```python
from build123d import *

# Parameters (mm, degrees)
SM_BASE_FLANGE_3_DEPTH = 50
SKETCH_14_R            = 6
SKETCH_14_R_2          = 1.5
CUT_EXTRUDE_1_DEPTH    = 69.26602376
SKETCH_15_R            = 2
CUT_EXTRUDE_2_DEPTH    = 94.257707456
FILLET_1_R             = 5


# Sheet-metal steps are written as plain solids
with BuildPart() as part:
    # 草图1 → 基体-法兰3 (new body)
    with BuildSketch(Plane(origin=(0, 0, 0), x_dir=(1, 0, 0), z_dir=(0, 1, 0))):
        with BuildLine():
            Line((-35.5, 34), (-35.5, 6))
            ThreePointArc((-35.5, 6), (-33.742640687, 1.757359313), (-29.5, 0))
            Line((-29.5, 0), (29.5, 0))
            ThreePointArc((29.5, 0), (33.742640687, 1.757359313), (35.5, 6))
            Line((35.5, 6), (35.5, 34))
            Line((35.5, 34), (31.5, 34))
            Line((31.5, 34), (31.5, 6))
            ThreePointArc((31.5, 6), (30.914213562, 4.585786438), (29.5, 4))
            Line((29.5, 4), (-29.5, 4))
            ThreePointArc((-29.5, 4), (-30.914213562, 4.585786438), (-31.5, 6))
            Line((-31.5, 6), (-31.5, 34))
            Line((-31.5, 34), (-35.5, 34))
        make_face()
    extrude(amount=SM_BASE_FLANGE_3_DEPTH)

    # 草图14 → 切除-拉伸1 (cut, through all)
    with BuildSketch(Plane(origin=(0, 0, -4), x_dir=(-1, 0, 0), z_dir=(0, 0, -1))):
        with Locations((0, 25)):
            Circle(SKETCH_14_R)
        with Locations((0, 37.5)):
            Circle(SKETCH_14_R_2)
        with Locations((12.5, 25)):
            Circle(SKETCH_14_R_2)
        with Locations((0, 12.5)):
            Circle(SKETCH_14_R_2)
        with Locations((-12.5, 25)):
            Circle(SKETCH_14_R_2)
    extrude(amount=-CUT_EXTRUDE_1_DEPTH, mode=Mode.SUBTRACT)

    # 草图15 → 切除-拉伸2 (cut, through all)
    with BuildSketch(Plane(origin=(35.5, 0, 0), x_dir=(0, 0, -1), z_dir=(1, 0, 0))):
        with Locations((15, 9)):
            Circle(SKETCH_15_R)
        with Locations((15, 41)):
            Circle(SKETCH_15_R)
        with Locations((27, 41)):
            Circle(SKETCH_15_R)
        with Locations((27, 9)):
            Circle(SKETCH_15_R)
    extrude(amount=-CUT_EXTRUDE_2_DEPTH, mode=Mode.SUBTRACT)

    # 圆角1
    fillet_1_edges = [part.edges().sort_by_distance(p)[0] for p in [
        (-33.5, 0, -34),
        (33.5, 0, -34),
        (-33.5, 50, -34),
        (33.5, 50, -34),
    ]]
    fillet(fillet_1_edges, radius=FILLET_1_R)


solid = part.part
```
Part model, mm, in its own coordinate system. A direction names the side the tool comes from. Round coordinates to 2 decimals unless told otherwise and drop trailing zeros. Write each loop counter-clockwise with the first axis right and the second up, starting at its lowest first coordinate (ties: lowest second). Pieces come first, ordered by that corner, then holes. Notation, with made-up numbers: M -28,-23.75 L 21,-23.75 A18 cw 21,-15.75 Z; hole C 32,32.5 d1. An arc over 180 degrees is marked long. Answer as CSV lines item,"result". Start each with the question number.
1) Which spindle directions (+Z, -Z, +X, -X, +Y, -Y) get a long thin tool onto all of the face, cutting with end or side? Do faces 4 (the face through (34, 25, -34)), 5 (the face through (-31.5, 25, -20)). Say none if no direction does.
2) Drill centre lines: L1, parallel to Y at x = 32.7, z = -15; L2, parallel to Y at x = 0, z = -2.7; L3, parallel to X at y = 27.5, z = -11. Where is each one in solid material? Low to high.
3) Mould opens along Z. For faces 1 (the face through (-33.789, 24.65, -1.804)), 2 (the face through (-33.472, 10.352, -13.526)), 3 (the face through (-35.5, 25, -20)) say: +Z half, -Z half, draft (parallel to the pull), parting line (faces both ways), or undercut.
4) Band-saw the part on A-A (z = -22). List the corners of the cut face in (x, y), then the cut area to 3 significant figures.
5) Band-saw the part on B-B (y = 9). List the corners of the cut face in (x, z), then the cut area to 3 significant figures.
6) Drop flat-ended pins along their axis: pin 1 (2.5 mm diameter, centred on x = 12.5, y = 25, fed in from +Z); pin 2 (1 mm diameter, centred on x = 4.5, y = 29, fed in from -Z). Give the stop position or say it passes through.
7) Band-saw the part on D-D (z = -27). List the corners of the cut face in (x, y).
8) Band-saw the part on C-C (y = 37.5). List the corners of the cut face in (x, z).
Worked out:
1,face 4,"-Z, +X, -X, +Y, -Y"
1,face 5,"-Z, +Y, -Y"
2,L1,"0 to 7, 11 to 39, 43 to 50"
2,L2,"0 to 11, 14 to 19, 31 to 36, 39 to 50"
2,L3,"-35.5 to -31.5, 31.5 to 35.5"
3,face 1,"+Z half"
3,face 2,"undercut"
3,face 3,"draft"
4,outline,"M -35.5,0 L -31.5,0 L -31.5,50 L -35.5,50 Z; M 31.5,0 L 35.5,0 L 35.5,50 L 31.5,50 Z"
4,area,"400 mm²"
5,outline,"M -35.5,-34 L -31.5,-34 L -31.5,-29 L -35.5,-29 Z; M -35.5,-25 L -31.5,-25 L -31.5,-17 L -35.5,-17 Z; M -35.5,-13 L -31.5,-13 L -31.5,-6 A2 cw -29.5,-4 L 29.5,-4 A2 cw 31.5,-6 L 31.5,-13 L 35.5,-13 L 35.5,-6 A6 ccw 29.5,0 L -29.5,0 A6 ccw -35.5,-6 Z; M 31.5,-34 L 35.5,-34 L 35.5,-29 L 31.5,-29 Z; M 31.5,-25 L 35.5,-25 L 35.5,-17 L 31.5,-17 Z"
5,area,"446 mm²"
6,pin 1,"through"
6,pin 2,"z = -4"
7,outline,"M -35.5,0 L -31.5,0 L -31.5,7 L -35.5,7 Z; M -35.5,11 L -31.5,11 L -31.5,39 L -35.5,39 Z; M -35.5,43 L -31.5,43 L -31.5,50 L -35.5,50 Z; M 31.5,0 L 35.5,0 L 35.5,7 L 31.5,7 Z; M 31.5,11 L 35.5,11 L 35.5,39 L 31.5,39 Z; M 31.5,43 L 35.5,43 L 35.5,50 L 31.5,50 Z"
8,outline,"M -35.5,-34 L -31.5,-34 L -31.5,-6 A2 cw -29.5,-4 L -1.5,-4 L -1.5,0 L -29.5,0 A6 ccw -35.5,-6 Z; M 1.5,-4 L 29.5,-4 A2 cw 31.5,-6 L 31.5,-34 L 35.5,-34 L 35.5,-6 A6 ccw 29.5,0 L 1.5,0 Z"
